from build123d import *

# Parameters (mm, degrees)
PAD_DEPTH    = 5
CHAMFER_SIZE = 2
FILLET_R     = 1.5
FILLET001_R  = 3


with BuildPart() as part:
    # Sketch → Pad (new body)
    with BuildSketch(Plane.XY):
        Polygon((0, 0), (0, 14), (24.1, 14), (24.1, 0), (22.1, 0), (19.1, 3.1), (22.1, 6.2), (22.1, 12), (2, 12), (2, 6.2), (5, 3.1), (2, 0), align=None)
    extrude(amount=PAD_DEPTH)

    # Chamfer
    chamfer_edges = [part.edges().sort_by_distance(p)[0] for p in [
        (5, 3.1, 2.5),
        (19.1, 3.1, 2.5),
    ]]
    chamfer(chamfer_edges, length=CHAMFER_SIZE)

    # Fillet
    fillet_edges = [part.edges().sort_by_distance(p)[0] for p in [
        (2, 12, 2.5),
        (22.1, 12, 2.5),
    ]]
    fillet(fillet_edges, radius=FILLET_R)

    # Fillet001
    fillet001_edges = [part.edges().sort_by_distance(p)[0] for p in [
        (0, 14, 2.5),
        (24.1, 14, 2.5),
    ]]
    fillet(fillet001_edges, radius=FILLET001_R)


solid = part.part
Model file for the job. Use its own axes, mm. A direction names the side the tool comes from. Give positions to 0.01 mm unless a question says otherwise; leave off trailing zeros. Loops run counter-clockwise (first coordinate to the right, second up) from the corner with the lowest first, then second, coordinate; pieces in that order, holes last.
Item 1: Drop a flat-ended pin along its axis: P1, Ø2.5, axis at x = 9, z = 2.5, coming from the -Y side. Give the stop position or say it passes through.
Check values:
P1: stops at y = 12
Item 2: Mould opens along Y. For faces 1 (the face through (23, 0, 2)), 2 (the face through (22.1, 8, 2)), 3 (the face through (12, 14, 2)) say: +Y half, -Y half, draft (parallel to the pull), parting line (faces both ways), or undercut.
Check values:
face 1: -Y half
face 2: undercut
face 3: +Y half
Item 3: Drill centre lines: line 1 along X through (y, z) = (9.25, 1.8); line 2 along X through (y, z) = (2.75, 1.3); line 3 along Y through (x, z) = (6.5, 4.25). Where is each one in solid material? Low to high.
Check values:
line 1: x = 0 to 2, 22.1 to 24.1
line 2: x = 0 to 3.61, 20.49 to 24.1
line 3: y = 12 to 14
Item 4: Slice it at C-C (z = 2.15). Write the cut outline in (x, y), plus the area to 3 significant figures.
Check values:
outline: (0, 0) - (2, 0) - (3.61, 1.66) - (3.61, 4.54) - (2, 6.2) - (2, 10.5) arc R1.5 cw to (3.5, 12) - (20.6, 12) arc R1.5 cw to (22.1, 10.5) - (22.1, 6.2) - (20.49, 4.54) - (20.49, 1.66) - (22.1, 0) - (24.1, 0) - (24.1, 11) arc R3 ccw to (21.1, 14) - (3, 14) arc R3 ccw to (0, 11) - close
area: 108 mm2
Item 5: Slice it at B-B (y = 2.25). Write the cut outline in (x, z).
Check values:
outline: (0, 0) - (3.61, 0) - (3.61, 5) - (0, 5) - close; (20.49, 0) - (24.1, 0) - (24.1, 5) - (20.49, 5) - close
Item 6: Slice it at A-A (y = 9.75). Write the cut outline in (x, z).
Check values:
outline: (0, 0) - (2, 0) - (2, 5) - (0, 5) - close; (22.1, 0) - (24.1, 0) - (24.1, 5) - (22.1, 5) - close
Item 7: Slice it at D-D (x = 20). Write the cut outline in (y, z), plus the area to 3 significant figures.
Check values:
outline: (12, 0) - (14, 0) - (14, 5) - (12, 5) - close
area: 10.0 mm2
Item 8: Which spindle directions (+Z, -Z, +X, -X, +Y, -Y) get a long thin tool onto all of the face, cutting with end or side? Do faces 4 (the face through (21.284, 5.357, 2.465)), 5 (the face through (0, 5, 2)), 6 (the face through (20.491, 3, 2)). Say none if no direction does.
Check values:
face 4: +Z, -Z
face 5: +Z, -Z, -X, +Y, -Y
face 6: +Z, -Z, -Y
